Verification items for the finished model (mm, model axes). A direction names the side the tool comes from. Give positions to 0.01 mm unless a question says otherwise; leave off trailing zeros. Loops run counter-clockwise (first coordinate to the right, second up) from the corner with the lowest first, then second, coordinate; pieces in that order, holes last. Notation, with made-up numbers: M -21,48.5 L -10,48.5 A31 cw -10,84.5 Z; hole C 59,3 d10. An arc over 180 degrees is marked long. Use a Markdown table: item, result.
from build123d import *

# Parameters (mm, degrees)
SKETCH1_W           = 38.1
SKETCH1_H           = 19.05
BOSS_EXTRUDE1_DEPTH = 18.5
BOSS_EXTRUDE3_DEPTH = 3.175
BOSS_EXTRUDE4_DEPTH = 18.5


with BuildPart() as part:
    # Sketch1 → Boss-Extrude1 (new body, symmetric)
    with BuildSketch(Plane(origin=(0, 0, 0), x_dir=(1, 0, 0), z_dir=(0, 1, 0))):
        with Locations((0, -34.925)):
            Rectangle(SKETCH1_W, SKETCH1_H)
    extrude(amount=BOSS_EXTRUDE1_DEPTH, both=True)

    # Sketch4 → Boss-Extrude3 (add, symmetric)
    with BuildSketch(Plane(origin=(0, 0, 0), x_dir=(1, 0, 0), z_dir=(0, 1, 0))):
        with BuildLine():
            Line((-19.05, -44.45), (-37.625792344, -103.364886448))
            ThreePointArc((-37.625792344, -103.364886448), (0, -110), (37.625792344, -103.364886448))
            Line((37.625792344, -103.364886448), (19.05, -44.45))
            Line((19.05, -44.45), (-19.05, -44.45))
        make_face()
    extrude(amount=BOSS_EXTRUDE3_DEPTH, both=True)

    # Sketch7 → Boss-Extrude4 (add, symmetric)
    with BuildSketch(Plane(origin=(0, 0, 0), x_dir=(1, 0, 0), z_dir=(0, 1, 0))):
        with BuildLine():
            Line((-29.987865037, -79.140475899), (-45.263719652, -127.589296997))
            ThreePointArc((-45.263719652, -127.589296997), (0, -135.380327319), (45.263719652, -127.589296997))
            Line((45.263719652, -127.589296997), (29.987865037, -79.140475899))
            ThreePointArc((29.987865037, -79.140475899), (0, -84.631477448), (-29.987865037, -79.140475899))
        make_face()
    extrude(amount=BOSS_EXTRUDE4_DEPTH, both=True)


solid = part.part
(1) Gauge pin test, flat ends, axial feed: P1, Ø12, axis at x = 19, y = 5.5, coming from the +Z side; P2, Ø4.5, axis at x = 5, y = -14.5, coming from the +Z side; P3, Ø5.5, axis at y = -6.5, z = 31, coming from the +X side. Record the tip position at first contact, or that the pin passes through.
Results below:
| item | result |
|---|---|
| P1 | z = 134.75 |
| P2 | z = 135.35 |
| P3 | x = 19.05 |
(2) Material ranges on line 1 (Z direction, x = -0.5, y = -14.5); line 2 (Y direction, x = -13.5, z = 48.5) (3 decimals); line 3 (Z direction, x = 4, y = -3.5), recorded low to high.
Results below:
| item | result |
|---|---|
| line 1 | 25.4 to 44.45, 84.63 to 135.38 |
| line 2 | -3.175 to 3.175 |
| line 3 | 25.4 to 44.45, 84.54 to 135.32 |
(3) Cross-section at A-A on y = 12.5. Record the cut outline in (x, z), then the cut area to 3 significant figures.
Results below:
| item | result |
|---|---|
| outline | M -45.26,127.59 L -29.99,79.14 A84.63 cw 29.99,79.14 L 45.26,127.59 A135.38 ccw Z; M -19.05,25.4 L 19.05,25.4 L 19.05,44.45 L -19.05,44.45 Z |
| area | 4,620 mm^2 |
(4) Cross-section at D-D on x = 9.5. Record the cut outline in (y, z) (3 decimals).
Results below:
| item | result |
|---|---|
| outline | M -18.5,25.4 L 18.5,25.4 L 18.5,44.45 L 3.175,44.45 L 3.175,84.097 L 18.5,84.097 L 18.5,135.047 L -18.5,135.047 L -18.5,84.097 L -3.175,84.097 L -3.175,44.45 L -18.5,44.45 Z |
(5) Draft check along Z on faces 5 (the cylindrical face through (-0.65, 0.26, 135.38)), 6 (the flat face through (0, 0, 25.4)), 7 (the flat face through (0, -3.175, 64)), 8 (the flat face through (19.05, 0, 35)). Enter one of: +Z half, -Z half, draft (parallel to the pull), parting line (faces both ways), or undercut.
Results below:
| item | result |
|---|---|
| face 5 | +Z half |
| face 6 | -Z half |
| face 7 | undercut |
| face 8 | draft |
(6) Cross-section at B-B on z = 91. Record the cut outline in (x, y) (3 decimals).
Results below:
| item | result |
|---|---|
| outline | M -33.727,-18.5 L 33.727,-18.5 L 33.727,18.5 L -33.727,18.5 Z |
(7) Cross-section at C-C on x = -21. Record the cut outline in (y, z) (3 decimals).
Results below:
| item | result |
|---|---|
| outline | M -18.5,81.985 L -3.175,81.985 L -3.175,50.635 L 3.175,50.635 L 3.175,81.985 L 18.5,81.985 L 18.5,133.742 L -18.5,133.742 Z |
(8) Set-up check for faces 1 (the cylindrical face through (0.43, 10.94, 84.63)), 2 (the flat face through (0, 11, 44.45)), 3 (the flat face through (-19.05, 0, 35)), 4 (the flat face through (0, -11, 44.45)): record each of +Z, -Z, +X, -X, +Y, -Y from which the full face is reachable in a straight line by a thin tool's end or side.
Results below:
| item | result |
|---|---|
| face 1 | +Y |
| face 2 | +X, -X, +Y |
| face 3 | -Z, -X, +Y, -Y |
| face 4 | +X, -X, -Y |
